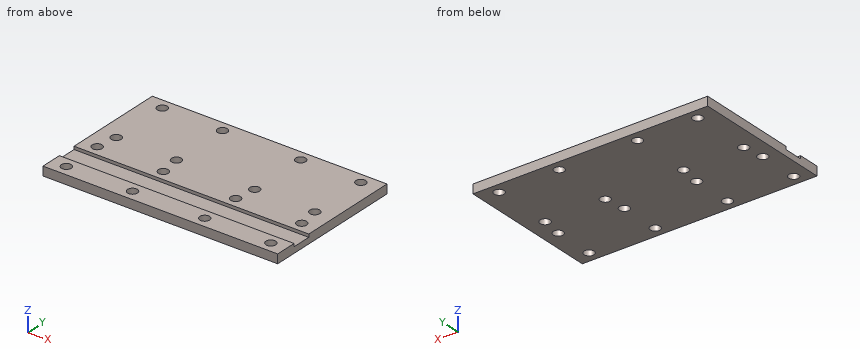
```python
from build123d import *

# Parameters (mm, degrees)
SKETCH_W     = 78
SKETCH_H     = 47.5
SKETCH_R     = 1.65
PAD_DEPTH    = 3
SKETCH001_W  = 105.620613
SKETCH001_H  = 6.4
POCKET_DEPTH = 1


with BuildPart() as part:
    # Sketch → Pad (new body)
    with BuildSketch(Plane.XY):
        with Locations((23, -10.25)):
            Rectangle(SKETCH_W, SKETCH_H)
        with Locations((-10, -10)):
            Circle(SKETCH_R, mode=Mode.SUBTRACT)
        with Locations((-10, 10)):
            Circle(SKETCH_R, mode=Mode.SUBTRACT)
        with Locations((10, 10)):
            Circle(SKETCH_R, mode=Mode.SUBTRACT)
        with Locations((10, -10)):
            Circle(SKETCH_R, mode=Mode.SUBTRACT)
        with Locations((-11, -17)):
            Circle(SKETCH_R, mode=Mode.SUBTRACT)
        with Locations((11, -17)):
            Circle(SKETCH_R, mode=Mode.SUBTRACT)
        with Locations((-11, -30.4)):
            Circle(SKETCH_R, mode=Mode.SUBTRACT)
        with Locations((11, -30.4)):
            Circle(SKETCH_R, mode=Mode.SUBTRACT)
        with Locations((56, -10)):
            Circle(SKETCH_R, mode=Mode.SUBTRACT)
        with Locations((56, 10)):
            Circle(SKETCH_R, mode=Mode.SUBTRACT)
        with Locations((36, 10)):
            Circle(SKETCH_R, mode=Mode.SUBTRACT)
        with Locations((36, -10)):
            Circle(SKETCH_R, mode=Mode.SUBTRACT)
        with Locations((35, -17)):
            Circle(SKETCH_R, mode=Mode.SUBTRACT)
        with Locations((35, -30.4)):
            Circle(SKETCH_R, mode=Mode.SUBTRACT)
        with Locations((57, -17)):
            Circle(SKETCH_R, mode=Mode.SUBTRACT)
        with Locations((57, -30.4)):
            Circle(SKETCH_R, mode=Mode.SUBTRACT)
    extrude(amount=PAD_DEPTH)

    # Sketch001 → Pocket (cut)
    with BuildSketch(Plane.XY.offset(3)):
        with Locations((22.581388, -23.7)):
            Rectangle(SKETCH001_W, SKETCH001_H)
    extrude(amount=-POCKET_DEPTH, mode=Mode.SUBTRACT)


solid = part.part
```
Geometry check sheet. Reference: the model listing, model coordinates, mm. Coordinates: 2 decimals unless noted, no trailing zeros. Loops run counter-clockwise (first coordinate to the right, second up) from the corner with the lowest first, then second, coordinate; pieces in that order, holes last.
Item 1: Thickness scan on line 1 (Y direction, x = 36, z = 1.6); line 2 (X direction, y = -8.5, z = 1.5); line 3 (Y direction, x = 9.5, z = 1.7). Record the ranges inside material, lowest first.
Item 2: Sectioned sample at A-A, the plane y = -17. Record the boundary of the cut face in (x, z).
Item 3: Sectioned sample at C-C, the plane x = -5. Record the boundary of the cut face in (y, z), then the cut area to 3 significant figures.
Item 4: Sectioned sample at B-B, the plane z = 1. Count the separate pieces of the cut face and the enclosed holes in it, then the cut area to 3 significant figures.
Item 5: Go/stop test with flat-tipped pins: pin 1 Ø5 at (x, y) = (24.5, -24) entering from +Z; pin 2 Ø2 at (x, y) = (56, -10) entering from -Z. Record where each tip stops, or that it passes through.
Check result:
1. line 1: y = -34 to -31.71, -29.09 to -18.31, -15.69 to -11.65, -8.35 to 8.35, 11.65 to 13.5
1. line 2: x = -16 to -10.69, -9.31 to 9.31, 10.69 to 35.31, 36.69 to 55.31, 56.69 to 62
1. line 3: y = -34 to -31.09, -29.71 to -17.69, -16.31 to -11.57, -8.43 to 8.43, 11.57 to 13.5
2. outline: (-16, 0) - (-12.65, 0) - (-12.65, 3) - (-16, 3) - close; (-9.35, 0) - (9.35, 0) - (9.35, 3) - (-9.35, 3) - close; (12.65, 0) - (33.35, 0) - (33.35, 3) - (12.65, 3) - close; (36.65, 0) - (55.35, 0) - (55.35, 3) - (36.65, 3) - close; (58.65, 0) - (62, 0) - (62, 3) - (58.65, 3) - close
3. outline: (-34, 0) - (13.5, 0) - (13.5, 3) - (-20.5, 3) - (-20.5, 2) - (-26.9, 2) - (-26.9, 3) - (-34, 3) - close
3. area: 136 mm2
4. separate pieces: 1
4. enclosed holes: 16
4. area: 3,570 mm2
5. pin 1: stops at z = 2
5. pin 2: passes through
